```python
from build123d import *

# Parameters (mm, degrees)
SKETCH1_R           = 2
BOSS_EXTRUDE1_DEPTH = 3
BOSS_EXTRUDE2_DEPTH = 3
CUT_EXTRUDE2_DEPTH  = 3
FILLET1_R           = 10
FILLET2_R           = 2


with BuildPart() as part:
    # Sketch1 → Boss-Extrude1 (new body)
    with BuildSketch(Plane(origin=(0, 0, 0), x_dir=(1, 0, 0), z_dir=(0, 1, 0))):
        with BuildLine():
            ThreePointArc((15.4216389, 2.828493148), (21.078493148, 2.8283611), (21.0783611, -2.828493148))
            ThreePointArc((21.0783611, -2.828493148), (0, -11.559147965), (-21.0783611, -2.828493148))
            ThreePointArc((-21.0783611, -2.828493148), (-21.078493148, 2.8283611), (-15.4216389, 2.828493148))
            ThreePointArc((-15.4216389, 2.828493148), (0, -3.559147965), (15.4216389, 2.828493148))
        make_face()
        with Locations((18.25, 0)):
            Circle(SKETCH1_R, mode=Mode.SUBTRACT)
        with Locations((-18.25, 0)):
            Circle(SKETCH1_R, mode=Mode.SUBTRACT)
    extrude(amount=BOSS_EXTRUDE1_DEPTH)

    # Sketch2 → Boss-Extrude2 (add)
    with BuildSketch(Plane(origin=(0, 3, 0), x_dir=(1, 0, 0), z_dir=(0, 1, 0))):
        with BuildLine():
            Line((-7.5, -10.600250197), (-7.5, -20.600250197))
            Line((-7.5, -20.600250197), (7.5, -20.600250197))
            Line((7.5, -20.600250197), (7.5, -10.600250197))
            ThreePointArc((7.5, -10.600250197), (0, -11.559147965), (-7.5, -10.600250197))
        make_face()
    extrude(amount=-BOSS_EXTRUDE2_DEPTH)

    # Sketch4 → Cut-Extrude2 (cut)
    with BuildSketch(Plane(origin=(0, 3, 0), x_dir=(1, 0, 0), z_dir=(0, 1, 0))):
        Polygon((-1.5, -20.600250197), (-1.5, -17.600250197), (-2.8, -17.600250197), (-2.8, -15.100250197), (-1.5, -15.100250197), (-1.5, -12.100250197), (-5, -12.100250197), (-5, -9.100250197), (5, -9.100250197), (5, -12.100250197), (1.5, -12.100250197), (1.5, -15.100250197), (2.8, -15.100250197), (2.8, -17.600250197), (1.5, -17.600250197), (1.5, -20.600250197), align=None)
    extrude(amount=-CUT_EXTRUDE2_DEPTH, mode=Mode.SUBTRACT)

    # Fillet1
    fillet1_edges = [part.edges().sort_by_distance(p)[0] for p in [
        (-7.5, 1.5, 10.600250197),
        (7.5, 1.5, 10.600250197),
    ]]
    fillet(fillet1_edges, radius=FILLET1_R)

    # Fillet2
    fillet2_edges = [part.edges().sort_by_distance(p)[0] for p in [
        (7.5, 1.5, 20.600250197),
        (-7.5, 1.5, 20.600250197),
    ]]
    fillet(fillet2_edges, radius=FILLET2_R)


solid = part.part
```
Design review of the part built by this model. Coordinates are the model's own, in mm. A direction names the side the tool comes from. Round coordinates to 2 decimals unless told otherwise and drop trailing zeros. Write each loop counter-clockwise with the first axis right and the second up, starting at its lowest first coordinate (ties: lowest second). Pieces come first, ordered by that corner, then holes. Notation, with made-up numbers: (8.5, -31) -> (50.5, -31) arc R16 ccw to (50.5, -19) -> close; hole circle Ø8 at (67.5, -28). An arc over 180 degrees is marked (long way). Write item = value, one per line. Start each with the question number.
1) Take a section at C-C, the plane x = 18.25. State the section outline as (y, z) points, plus the area to 3 significant figures.
2) Clearance check with flat-ended pins moving along their axes: pin 1 (0.9 mm diameter, centred on y = 1.5, z = 18, fed in from +X); pin 2 (0.9 mm diameter, centred on x = -4, y = 1.5, fed in from -Z); pin 3 (1.5 mm diameter, centred on y = 2, z = 14.5, fed in from -X). State where each tip first meets the part, or that it passes through.
3) Take a section at A-A, the plane y = 2.25. Count the separate pieces of the cut face and the enclosed holes in it, plus the area to 3 significant figures.
4) Mouldability with a two-part tool opening along X and no side actions: class faces 1 (the face through (-2, 2, 15.1)), 2 (the face through (9.058, 1.479, 12.147)), 3 (the face through (0, 0, 8)), 4 (the face through (3, 2, 12.1)) as +X half, -X half, draft (parallel to the pull), parting line (faces both ways), or undercut.
5) Tool access review of faces 5 (the face through (2, 2, 17.6)), 6 (the face through (0, 3, 8)), 7 (the face through (1.5, 2, 14)): name each direction out of +Z, -Z, +X, -X, +Y, -Y from which nothing blocks a thin tool from reaching the whole face with its end or side.
6) Wall thickness on probe 1 along X at (y, z) = (2.2, 0); probe 2 along X at (y, z) = (0.8, -0.75); probe 3 along Z at (x, y) = (-18.25, 1.5): over which ranges is each line inside the solid? List them lowest first. Write a range as from..to.
7) Take a section at B-B, the plane z = 15.75. State the section outline as (x, y) points.
8) Take a section at D-D, the plane z = -1. State the section outline as (x, y) points.
Results list:
q1.outline = (0, -4) -> (3, -4) -> (3, -2) -> (0, -2) -> close; (0, 2) -> (3, 2) -> (3, 5.32) -> (0, 5.32) -> close
q1.area = 16.0 mm²
q2.pin_1 = 7.5
q2.pin_2 = 3.1
q2.pin_3 = -8.23
q3.separate_pieces = 1
q3.enclosed_holes = 2
q3.area = 442 mm²
q4.face_1 = undercut
q4.face_2 = +X half
q4.face_3 = draft
q4.face_4 = undercut
q5.face_5 = +Y, -Y
q5.face_6 = +Z, -Z, +X, -X, +Y
q5.face_7 = +Z, +Y, -Y
q6.probe_1 = -22.25..-20.25, -16.25..-11.94, 11.94..16.25, 20.25..22.25
q6.probe_2 = -22.18..-20.1, -16.4..-13.02, 13.02..16.4, 20.1..22.18
q6.probe_3 = -4..-2, 2..5.32
q7.outline = (-7.66, 0) -> (-2.8, 0) -> (-2.8, 3) -> (-7.66, 3) -> close; (2.8, 0) -> (7.66, 0) -> (7.66, 3) -> (2.8, 3) -> close
q8.outline = (-22.12, 0) -> (-19.98, 0) -> (-19.98, 3) -> (-22.12, 3) -> close; (-16.52, 0) -> (-13.34, 0) -> (-13.34, 3) -> (-16.52, 3) -> close; (13.34, 0) -> (16.52, 0) -> (16.52, 3) -> (13.34, 3) -> close; (19.98, 0) -> (22.12, 0) -> (22.12, 3) -> (19.98, 3) -> close
